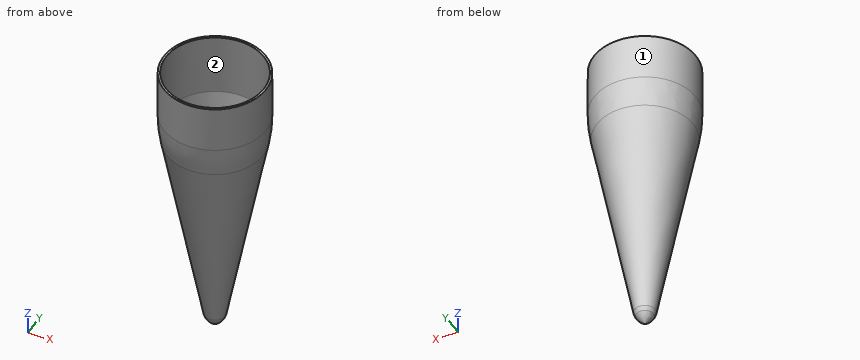
from build123d import *

# Parameters (mm, degrees)
FILLET1_R = 254
FILLET2_R = 20.32


# Read off the part's stored shape, not the designer's step: Shell1
with BuildPart() as part:
    # Sketch3 → Revolve1 (revolve)
    with BuildSketch(Plane(origin=(0, 0, 0), x_dir=(1, 0, 0), z_dir=(0, 1, 0))):
        with BuildLine():
            Line((79.375, 0), (79.375, 97.566452781))
            Line((79.375, 97.566452781), (15.414998094, 435.593871211))
            ThreePointArc((15.414998094, 435.593871211), (9.023509201, 445.178624931), (0, 452.340671834))
            Line((0, 452.340671834), (0, 431.8))
            Line((0, 431.8), (0, 0))
            Line((0, 0), (79.375, 0))
        make_face()
    revolve(axis=Axis((0, 0, -20.618215306), (0, 0, -1)))

    # Shell1 outline → Shell1 (revolve, cut)
    with BuildSketch(Plane.XZ):
        with BuildLine():
            add(Edge.make_bspline(
                [(0, -448.485192633), (8.107967388, -443.274294187), (12.248008898, -434.570694124)],
                knots=[5.283607214, 5.283607214, 5.283607214, 5.839190446, 5.839190446, 5.839190446], degree=2, weights=[1, 0.961663394, 1]))
            Line((12.248008898, -434.570694124), (76.073, -97.256805277))
            Line((76.073, -97.256805277), (76.073, 0))
            Line((76.073, 0), (0, 0))
            Line((0, 0), (0, -448.485192633))
        make_face()
    revolve(axis=Axis((0, 0, 0), (0, 0, 1)), mode=Mode.SUBTRACT)

    # Fillet1
    fillet1_edges = [part.edges().sort_by_distance(p)[0] for p in [
        (-79.375, 0, -97.566452781),
    ]]
    fillet(fillet1_edges, radius=FILLET1_R)

    # Fillet2
    fillet2_edges = [part.edges().sort_by_distance(p)[0] for p in [
        (-15.414998094, 0, -435.593871211),
    ]]
    fillet(fillet2_edges, radius=FILLET2_R)


solid = part.part
Could you check a few things on this model? Use its own coordinates, in mm. Face numbers are marked on the shaded views. Coordinates: 2 decimals unless noted, no trailing zeros. Order: outer loops, then holes, each group sorted by start corner. A loop starts at its lowest first (then second) coordinate and runs counter-clockwise, first axis right, second up.
Q1. Suppose I cut it at A-A on z = -400.5. Please give me the cut outline in (x, y), and give its area (3 significant figures).
Q2. Suppose I cut it at B-B on z = -245.5. Please give me the cut outline in (x, y).
Q3. Thinking about a two-plate mould opening in Y: for the marked faces 1 and 2, which applies, released by +Y, released by -Y, zero draft, split by the parting line, or undercut?
Q4. Will these pins go through, and if not, where does the flat tip stop? pin 1 (12 mm diameter, centred on x = 29.5, z = -284.5, fed in from -Y); pin 2 (12 mm diameter, centred on y = 5, z = -64, fed in from +X) (3 decimals); pin 3 (8 mm diameter, centred on x = 19.5, z = -330.5, fed in from +Y); pin 4 (12 mm diameter, centred on x = -63, z = -96, fed in from +Y).
Q5. Please list where these lines run through material, in increasing order: L1, parallel to Y at x = 0, z = -26.5 (3 decimals); L2, parallel to X at y = 29, z = -189; L3, parallel to Y at x = 2.5, z = -362.
Answer:
1. outline: circle Ø44.11 at (0, 0); hole circle Ø37.39 at (0, 0)
1. area: 430 mm2
2. outline: circle Ø102.77 at (0, 0); hole circle Ø96.05 at (0, 0)
3. face 1: split by the parting line
3. face 2: undercut
4. pin 1: stops at y = -37.43
4. pin 2: stops at x = 79.375
4. pin 3: stops at y = 31.89
4. pin 4: stops at y = 53.87
5. L1: y = -79.375 to -76.073, 76.073 to 79.375
5. L2: x = -54.88 to -51.05, 51.05 to 54.88
5. L3: y = -29.23 to -25.86, 25.86 to 29.23
